Geometry check sheet. Reference: the model listing, model coordinates, mm. Face numbers are marked on the shaded views. A direction names the side the tool comes from. Round coordinates to 2 decimals unless told otherwise and drop trailing zeros. Loops run counter-clockwise (first coordinate to the right, second up) from the corner with the lowest first, then second, coordinate; pieces in that order, holes last. Notation, with made-up numbers: (-5.5, -24.75) -> (47.5, -24.75) arc R14 cw to (47.5, -16.75) -> close; hole circle Ø9 at (39.25, -1.5). An arc over 180 degrees is marked (long way). Use one line per item in the form item = value.
from build123d import *

# Parameters (mm, degrees)
F0_R   = 3.1877
F0_R_2 = 2.0193


with BuildPart() as f2:
    # F2: sweep along a path in F1
    with BuildLine(Plane.XZ) as f2_path:
        Line((0, 0), (27.655674, 0))
        ThreePointArc((27.655674, 0), (32.302863, 1.924929), (34.227792, 6.572118))
        Line((34.227792, 6.572118), (34.227792, 19.272118))
        ThreePointArc((34.227792, 19.272118), (36.092292, 23.773419), (40.593592, 25.637919))
        Line((40.593592, 25.637919), (56.098651, 25.637919))
    # F0 (on Right) → F2 (sweep)
    with BuildSketch(Plane.YZ):
        Circle(F0_R)
        Circle(F0_R_2, mode=Mode.SUBTRACT)
    sweep(path=f2_path.line)


solid = f2.part
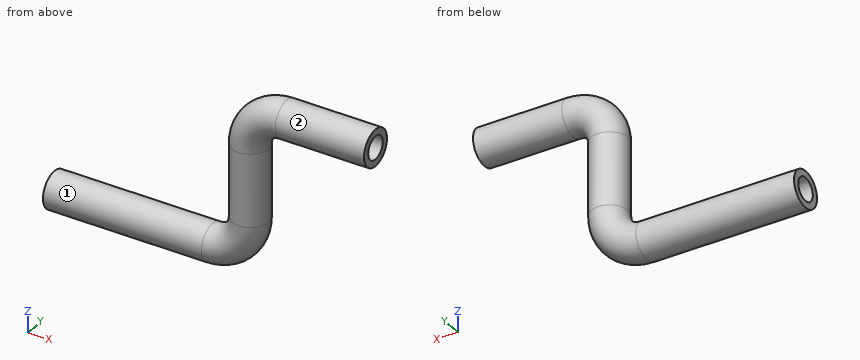
1. Gauge pin test, flat ends, axial feed: pin 1 (3 mm diameter, centred on x = 30, z = 18, fed in from -Y); pin 2 (8 mm diameter, centred on x = 38.5, z = 15, fed in from -Y); pin 3 (1 mm diameter, centred on x = 24.5, y = 2, fed in from +Z). Record the tip position at first contact, or that the pin passes through.
Return value:
pin_1 = -1.65
pin_2 = -3.18
pin_3 = 2.81
2. Material ranges on line 1 along Z through (x, y) = (15, 0); line 2 along X through (y, z) = (-0.5, 5); line 3 along X through (y, z) = (0.75, 13), recorded low to high.
Return value:
line_1 = -3.19 to -2.02, 2.02 to 3.19
line_2 = 30.7 to 32, 36.04 to 37.25
line_3 = 31.13 to 32.35, 36.1 to 37.33
3. Section check A-A (x = 43.5). Record the boundary of the cut face in (y, z).
Return value:
outline = circle Ø6.38 at (0, 25.64); hole circle Ø4.04 at (0, 25.64)
4. Tool access check on the marked faces 1 and 2. Record the directions out of +Z, -Z, +X, -X, +Y, -Y that give a thin tool (end or side, any length) a straight path to the whole face; none if there is none.
Return value:
face_1 = -X
face_2 = +X
